Geometry: final body of the model. Coordinates: model frame, mm. Round coordinates to 2 decimals unless told otherwise and drop trailing zeros. Order: outer loops, then holes, each group sorted by start corner. A loop starts at its lowest first (then second) coordinate and runs counter-clockwise, first axis right, second up. Notation, with made-up numbers: (-36.5, 6.25) -> (12.5, 6.25) arc R23 cw to (12.5, 25.25) -> close; hole circle Ø9 at (41.25, 64.25). An arc over 180 degrees is marked (long way). Put each result on its own line as item: value.
```python
from build123d import *

# Parameters (mm, degrees)
SKETCH1_R            = 36.5125
SKETCH1_R_2          = 17.4879
BOSS_EXTRUDE1_DEPTH  = 9.525
SKETCH2_R            = 17.4879
SKETCH2_R_2          = 12.7
BOSS_EXTRUDE2_DEPTH  = 9.525
SKETCH3_R            = 2.0193
CUT_EXTRUDE1_DEPTH   = 56.038421239
SKETCH4_W            = 4.7625
SKETCH4_H            = 9.525
CUT_EXTRUDE2_START   = -12.7
SKETCH5_R            = 2.4892
CUT_EXTRUDE2_DEPTH   = 12.7
CIRPATTERN1_COUNT    = 10
SPLIT1_START         = -9.525
SPLIT1_OUTLINE_R     = 36.5125
SPLIT1_OUTLINE_R_2   = 2.4892
SPLIT1_OUTLINE_R_3   = 12.7
SPLIT1_DEPTH         = 12.7
SPLIT1_START_2       = -6.35
SPLIT1_2_OUTLINE_R   = 31.75
SPLIT1_2_OUTLINE_R_2 = 2.4892
SPLIT1_2_OUTLINE_R_3 = 12.7
SPLIT1_2_DEPTH       = 6.35
SPLIT1_3_OUTLINE_R   = 31.75
SPLIT1_3_OUTLINE_R_2 = 2.4892
SPLIT1_3_OUTLINE_R_3 = 17.4879
SPLIT1_3_DEPTH       = 3.175
SPLIT1_4_OUTLINE_R   = 36.5125
SPLIT1_4_OUTLINE_R_2 = 2.4892
SPLIT1_4_OUTLINE_R_3 = 12.7
SPLIT1_4_DEPTH       = 3.175


# Read off the part's stored shape, not the designer's step: Split1
with BuildPart() as part:
    # Sketch1 → Boss-Extrude1 (new, symmetric)
    with BuildSketch(Plane(origin=(0, 0, 0), x_dir=(1, 0, 0), z_dir=(0, 1, 0))):
        with Locations(Location((0, 0, 0), (0, 0, 90))):
            Circle(SKETCH1_R)
        with Locations(Location((0, 0, 0), (0, 0, 90))):
            Circle(SKETCH1_R_2, mode=Mode.SUBTRACT)
    extrude(amount=BOSS_EXTRUDE1_DEPTH, both=True)

    # Sketch2 → Boss-Extrude2 (add)
    with BuildSketch(Plane.XZ.offset(9.525)):
        with Locations(Location((0, 0, 0), (0, 0, 270))):
            Circle(SKETCH2_R)
        with Locations(Location((0, 0, 0), (0, 0, 270))):
            Circle(SKETCH2_R_2, mode=Mode.SUBTRACT)
    extrude(amount=-BOSS_EXTRUDE2_DEPTH)

    # Sketch3 → Cut-Extrude1 (cut, through all)
    with BuildSketch(Plane.XZ.offset(9.525)):
        with Locations(Location((0, 21.2725, 0), (0, 0, 270))):
            Circle(SKETCH3_R)
    cut_extrude1 = extrude(amount=-CUT_EXTRUDE1_DEPTH, mode=Mode.SUBTRACT)

    # Sketch4 → Cut-Revolve1 (revolve, cut)
    with BuildSketch(Plane(origin=(0, 0, 0), x_dir=(0, 0, -1), z_dir=(1, 0, 0)), mode=Mode.PRIVATE) as cut_revolve1_sk:
        with Locations((-34.13125, -1.5875)):
            Rectangle(SKETCH4_W, SKETCH4_H)
    revolve(cut_revolve1_sk.sketch.rotate(Axis((0, 0, 0), (0, 1, 0)), 180), axis=Axis((0, 0, 0), (0, 1, 0)), mode=Mode.SUBTRACT)

    # Sketch5 → Cut-Extrude2 (cut)
    with BuildSketch(Plane.XZ.offset(9.525).offset(CUT_EXTRUDE2_START)):
        with Locations(Location((0, 21.2725, 0), (0, 0, 270))):
            Circle(SKETCH5_R)
    cut_extrude2 = extrude(amount=CUT_EXTRUDE2_DEPTH, mode=Mode.SUBTRACT)

    # CirPattern1: Cut-Extrude1, Cut-Extrude2 ×10 about axis
    cirpattern1_axis = Axis((0, 0, 0), (0, 1, 0))
    add([cut_extrude1.rotate(cirpattern1_axis, i * 360 / CIRPATTERN1_COUNT) for i in range(1, CIRPATTERN1_COUNT)], mode=Mode.SUBTRACT)
    add([cut_extrude2.rotate(cirpattern1_axis, i * 360 / CIRPATTERN1_COUNT) for i in range(1, CIRPATTERN1_COUNT)], mode=Mode.SUBTRACT)

    # Split1 outline → Split1 (cut)
    with BuildSketch(Plane(origin=(0, 0, 0), x_dir=(1, 0, 0), z_dir=(0, 1, 0)).offset(SPLIT1_START)):
        Circle(SPLIT1_OUTLINE_R)
        with Locations((0, 21.2725)):
            Circle(SPLIT1_OUTLINE_R_2, mode=Mode.SUBTRACT)
        with Locations((-20.231349743, -6.573564013)):
            Circle(SPLIT1_OUTLINE_R_2, mode=Mode.SUBTRACT)
        with Locations((-12.503661779, -17.209814013)):
            Circle(SPLIT1_OUTLINE_R_2, mode=Mode.SUBTRACT)
        with Locations((0, -21.2725)):
            Circle(SPLIT1_OUTLINE_R_2, mode=Mode.SUBTRACT)
        with Locations((12.503661779, -17.209814013)):
            Circle(SPLIT1_OUTLINE_R_2, mode=Mode.SUBTRACT)
        with Locations((20.231349743, -6.573564013)):
            Circle(SPLIT1_OUTLINE_R_2, mode=Mode.SUBTRACT)
        with Locations((-20.231349743, 6.573564013)):
            Circle(SPLIT1_OUTLINE_R_2, mode=Mode.SUBTRACT)
        with Locations((-12.503661779, 17.209814013)):
            Circle(SPLIT1_OUTLINE_R_2, mode=Mode.SUBTRACT)
        with Locations((12.503661779, 17.209814013)):
            Circle(SPLIT1_OUTLINE_R_2, mode=Mode.SUBTRACT)
        with Locations((20.231349743, 6.573564013)):
            Circle(SPLIT1_OUTLINE_R_2, mode=Mode.SUBTRACT)
        Circle(SPLIT1_OUTLINE_R_3, mode=Mode.SUBTRACT)
    extrude(amount=SPLIT1_DEPTH, mode=Mode.SUBTRACT)


with BuildPart() as body_2:
    # Split1 2 outline → Split1 2 (new body)
    with BuildSketch(Plane(origin=(0, 0, 0), x_dir=(1, 0, 0), z_dir=(0, 1, 0)).offset(SPLIT1_START_2)):
        Circle(SPLIT1_2_OUTLINE_R)
        with Locations((-12.503661779, -17.209814013)):
            Circle(SPLIT1_2_OUTLINE_R_2, mode=Mode.SUBTRACT)
        with Locations((-20.231349743, -6.573564013)):
            Circle(SPLIT1_2_OUTLINE_R_2, mode=Mode.SUBTRACT)
        with Locations((0, -21.2725)):
            Circle(SPLIT1_2_OUTLINE_R_2, mode=Mode.SUBTRACT)
        with Locations((12.503661779, -17.209814013)):
            Circle(SPLIT1_2_OUTLINE_R_2, mode=Mode.SUBTRACT)
        with Locations((20.231349743, -6.573564013)):
            Circle(SPLIT1_2_OUTLINE_R_2, mode=Mode.SUBTRACT)
        with Locations((-20.231349743, 6.573564013)):
            Circle(SPLIT1_2_OUTLINE_R_2, mode=Mode.SUBTRACT)
        with Locations((-12.503661779, 17.209814013)):
            Circle(SPLIT1_2_OUTLINE_R_2, mode=Mode.SUBTRACT)
        Circle(SPLIT1_2_OUTLINE_R_3, mode=Mode.SUBTRACT)
        with Locations((20.231349743, 6.573564013)):
            Circle(SPLIT1_2_OUTLINE_R_2, mode=Mode.SUBTRACT)
        with Locations((0, 21.2725)):
            Circle(SPLIT1_2_OUTLINE_R_2, mode=Mode.SUBTRACT)
        with Locations((12.503661779, 17.209814013)):
            Circle(SPLIT1_2_OUTLINE_R_2, mode=Mode.SUBTRACT)
    extrude(amount=SPLIT1_2_DEPTH)


with BuildPart() as body_3:
    # Split1 3 outline → Split1 3 (new body)
    with BuildSketch(Plane(origin=(0, 0, 0), x_dir=(1, 0, 0), z_dir=(0, 1, 0))):
        Circle(SPLIT1_3_OUTLINE_R)
        with Locations((-12.503661779, -17.209814013)):
            Circle(SPLIT1_3_OUTLINE_R_2, mode=Mode.SUBTRACT)
        with Locations((-20.231349743, -6.573564013)):
            Circle(SPLIT1_3_OUTLINE_R_2, mode=Mode.SUBTRACT)
        with Locations((0, -21.2725)):
            Circle(SPLIT1_3_OUTLINE_R_2, mode=Mode.SUBTRACT)
        with Locations((12.503661779, -17.209814013)):
            Circle(SPLIT1_3_OUTLINE_R_2, mode=Mode.SUBTRACT)
        with Locations((20.231349743, -6.573564013)):
            Circle(SPLIT1_3_OUTLINE_R_2, mode=Mode.SUBTRACT)
        with Locations((-20.231349743, 6.573564013)):
            Circle(SPLIT1_3_OUTLINE_R_2, mode=Mode.SUBTRACT)
        with Locations((-12.503661779, 17.209814013)):
            Circle(SPLIT1_3_OUTLINE_R_2, mode=Mode.SUBTRACT)
        Circle(SPLIT1_3_OUTLINE_R_3, mode=Mode.SUBTRACT)
        with Locations((20.231349743, 6.573564013)):
            Circle(SPLIT1_3_OUTLINE_R_2, mode=Mode.SUBTRACT)
        with Locations((0, 21.2725)):
            Circle(SPLIT1_3_OUTLINE_R_2, mode=Mode.SUBTRACT)
        with Locations((12.503661779, 17.209814013)):
            Circle(SPLIT1_3_OUTLINE_R_2, mode=Mode.SUBTRACT)
    extrude(amount=SPLIT1_3_DEPTH)


with BuildPart() as body_4:
    # Split1 4 outline → Split1 4 (new body)
    with BuildSketch(Plane(origin=(0, 0, 0), x_dir=(1, 0, 0), z_dir=(0, 1, 0)).offset(SPLIT1_START)):
        Circle(SPLIT1_4_OUTLINE_R)
        with Locations((-20.231349743, -6.573564013)):
            Circle(SPLIT1_4_OUTLINE_R_2, mode=Mode.SUBTRACT)
        with Locations((-12.503661779, -17.209814013)):
            Circle(SPLIT1_4_OUTLINE_R_2, mode=Mode.SUBTRACT)
        with Locations((0, -21.2725)):
            Circle(SPLIT1_4_OUTLINE_R_2, mode=Mode.SUBTRACT)
        with Locations((12.503661779, -17.209814013)):
            Circle(SPLIT1_4_OUTLINE_R_2, mode=Mode.SUBTRACT)
        with Locations((20.231349743, -6.573564013)):
            Circle(SPLIT1_4_OUTLINE_R_2, mode=Mode.SUBTRACT)
        with Locations((-20.231349743, 6.573564013)):
            Circle(SPLIT1_4_OUTLINE_R_2, mode=Mode.SUBTRACT)
        with Locations((-12.503661779, 17.209814013)):
            Circle(SPLIT1_4_OUTLINE_R_2, mode=Mode.SUBTRACT)
        Circle(SPLIT1_4_OUTLINE_R_3, mode=Mode.SUBTRACT)
        with Locations((12.503661779, 17.209814013)):
            Circle(SPLIT1_4_OUTLINE_R_2, mode=Mode.SUBTRACT)
        with Locations((20.231349743, 6.573564013)):
            Circle(SPLIT1_4_OUTLINE_R_2, mode=Mode.SUBTRACT)
        with Locations((0, 21.2725)):
            Circle(SPLIT1_4_OUTLINE_R_2, mode=Mode.SUBTRACT)
    extrude(amount=SPLIT1_4_DEPTH)


solid = part.part
```
1. Cut plane C-C on y = 5.75. State how many separate pieces and enclosed holes the cut face has, and give its area (3 significant figures).
Ans:
separate pieces: 1
enclosed holes: 11
area: 3,100 mm²
2. Cut plane A-A on x = 0. Return loops of the section in (y, z) (1 decimal).
Ans:
outline: (3.2, -36.5) -> (9.5, -36.5) -> (9.5, -23.3) -> (3.2, -23.3) -> close; (3.2, -19.3) -> (9.5, -19.3) -> (9.5, -17.5) -> (3.2, -17.5) -> close; (3.2, 17.5) -> (9.5, 17.5) -> (9.5, 19.3) -> (3.2, 19.3) -> close; (3.2, 23.3) -> (9.5, 23.3) -> (9.5, 36.5) -> (3.2, 36.5) -> close
3. Cut plane D-D on x = 20.5. Return loops of the section in (y, z) (3 decimals).
Ans:
outline: (3.175, -30.214) -> (9.525, -30.214) -> (9.525, -8.575) -> (3.175, -8.575) -> close; (3.175, -4.572) -> (9.525, -4.572) -> (9.525, 4.572) -> (3.175, 4.572) -> close; (3.175, 8.575) -> (9.525, 8.575) -> (9.525, 30.214) -> (3.175, 30.214) -> close
4. Draft query along X for faces 1 (the face through (18.59, 6.31, 5.4)), 2 (the face through (16, 9.525, 9)), 3 (the face through (-10.967, 6.394, -34.826)). Return one class per face: +X half, -X half, draft (parallel to the pull), parting line (faces both ways), or undercut.
Ans:
face 1: undercut
face 2: draft
face 3: parting line
5. Material intervals for probe 1 along X at (y, z) = (7.25, 19); probe 2 along X at (y, z) = (6.5, -7); probe 3 along Z at (x, y) = (-18.5, 8), sorted ascending.
Ans:
probe 1: -31.18 to -13.44, -11.57 to 11.57, 13.44 to 31.18
probe 2: -35.84 to -22.21, -18.26 to -16.03, 16.03 to 18.26, 22.21 to 35.84
probe 3: -31.48 to -7.61, -5.53 to 5.53, 7.61 to 31.48
6. Contact query for flat-ended pins moving along their axis: P1, Ø2.5, axis at x = 0, z = 21.27, coming from the +Y side; P2, Ø1, axis at x = 19.5, y = 6, coming from the +Z side; P3, Ø1.5, axis at x = -10.5, y = 8.5, coming from the +Z side; P4, Ø3, axis at x = 19.5, y = 6.5, coming from the +Z side. Output: stop coordinate, or through.
Ans:
P1: through
P2: z = 31.18
P3: z = 35.19
P4: z = 31.77
7. Cut plane B-B on z = 0. Return loops of the section in (x, y) (1 decimal).
Ans:
outline: (-36.5, 3.2) -> (-17.5, 3.2) -> (-17.5, 9.5) -> (-36.5, 9.5) -> close; (17.5, 3.2) -> (36.5, 3.2) -> (36.5, 9.5) -> (17.5, 9.5) -> close
